Can you work these out from the model? Positions are in its coordinate system, mm. Face numbers are marked on the shaded views. Coordinates: 2 decimals unless noted, no trailing zeros. Order: outer loops, then holes, each group sorted by start corner. A loop starts at its lowest first (then second) coordinate and runs counter-clockwise, first axis right, second up. Notation, with made-up numbers: (-19, 47.5) -> (6, 47.5) arc R22 cw to (6, 64.5) -> close; hole circle Ø7 at (83.25, -12.5). An arc over 180 degrees is marked (long way). Return JSON: item names as keys, results as strings. Group by question number.
1) If we section it at C-C, the plane y = 7.25: Please give me the cut outline in (x, z) (3 decimals).
2) Thinking about a two-plate mould opening in Z: for the marked faces 1 and 2, which applies, +Z half, -Z half, draft (parallel to the pull), parting line (faces both ways), or undercut?
3) If I drill on probe 1 along Y at (x, z) = (-45.5, -2); probe 2 along Z at (x, y) = (-39, -1); probe 3 along Z at (x, y) = (-16, 0), over which ranges is the centre line in solid material (lowest first)? Write a range as from..to.
4) If we section it at B-B, the plane x = -43: Please give me the cut outline in (y, z), then the cut area to 3 significant figures.
5) For pin 1 (2 mm diameter, centred on y = -0.5, z = 1.5, fed in from +X); pin 2 (6 mm diameter, centred on x = -14, y = -0.5, fed in from -Z); pin 3 (1.5 mm diameter, centred on y = 2, z = -3, fed in from -X), each with a flat end and sliding along its axis, tell me the tip position at first contact or that it passes through.
from build123d import *

# Parameters (mm, degrees)
REVOLVE1_ANGLE                  = 67
BOSS_EXTRUDE1_REACH             = 76.037
BOSS_EXTRUDE1_END_RADIUS        = 72.791303716
BOSS_EXTRUDE1_DIRECTION_2_DEPTH = 4.5
BOSS_EXTRUDE2_DEPTH             = 4
BOSS_EXTRUDE3_DEPTH             = 1.35
CHAMFER1_SIZE                   = 0.5
SKETCH5_R                       = 1.475
BOSS_EXTRUDE4_DEPTH             = 7.1
SKETCH6_R                       = 3
BOSS_EXTRUDE5_DEPTH             = 3
BOSS_EXTRUDE5_TAPER             = 11
CHAMFER2_SIZE                   = 0.5
CHAMFER2_SIZE_2                 = 0.632256576


with BuildPart() as part:
    # Sketch1 → Revolve1 (revolve, symmetric)
    with BuildSketch(Plane.XY) as revolve1_sk:
        with BuildLine():
            Line((-60, 5), (-60.791303716, 5))
            Line((-60.791303716, 5), (-60.791303716, 6))
            Line((-60.791303716, 6), (-57.791303716, 6))
            Line((-57.791303716, 6), (-57.791303716, -6))
            Line((-57.791303716, -6), (-60.791303716, -6))
            Line((-60.791303716, -6), (-60.791303716, -5))
            Line((-60.791303716, -5), (-60, -5))
            ThreePointArc((-60, -5), (-59.791303716, 0), (-60, 5))
        make_face()
    revolve(axis=Axis((15, 24.442446043, 0), (0, -1, 0)), revolution_arc=REVOLVE1_ANGLE / 2)
    revolve(revolve1_sk.sketch, axis=Axis((15, 24.442446043, 0), (0, 1, 0)), revolution_arc=REVOLVE1_ANGLE / 2)

    # Boss-Extrude1: up to this cylinder (the profile starts inside it)
    boss_extrude1_end = Plane(origin=(15, 0, 0), z_dir=(0, 1, 0)) * Cylinder(BOSS_EXTRUDE1_END_RADIUS, 298.656607431, mode=Mode.PRIVATE)
    # Sketch2 → Boss-Extrude1 (add, up to the surface)
    with BuildSketch(Plane(origin=(0, 0, 0), x_dir=(0, 0, -1), z_dir=(1, 0, 0)), mode=Mode.PRIVATE) as boss_extrude1_sk1:
        with BuildLine():
            Line((2.75, 1.35), (-2.75, 1.35))
            ThreePointArc((-2.75, 1.35), (-2.926776695, 1.276776695), (-3, 1.1))
            Line((-3, 1.1), (-3, 1))
            ThreePointArc((-3, 1), (-2.926776695, 0.823223305), (-2.75, 0.75))
            Line((-2.75, 0.75), (-1.75, 0.75))
            ThreePointArc((-1.75, 0.75), (-1.573223305, 0.676776695), (-1.5, 0.5))
            Line((-1.5, 0.5), (-1.5, -0.5))
            ThreePointArc((-1.5, -0.5), (-1.573223305, -0.676776695), (-1.75, -0.75))
            Line((-1.75, -0.75), (-2.75, -0.75))
            ThreePointArc((-2.75, -0.75), (-2.926776695, -0.823223305), (-3, -1))
            Line((-3, -1), (-3, -1.1))
            ThreePointArc((-3, -1.1), (-2.926776695, -1.276776695), (-2.75, -1.35))
            Line((-2.75, -1.35), (2.75, -1.35))
            ThreePointArc((2.75, -1.35), (2.926776695, -1.276776695), (3, -1.1))
            Line((3, -1.1), (3, -1))
            ThreePointArc((3, -1), (2.926776695, -0.823223305), (2.75, -0.75))
            Line((2.75, -0.75), (1.75, -0.75))
            ThreePointArc((1.75, -0.75), (1.573223305, -0.676776695), (1.5, -0.5))
            Line((1.5, -0.5), (1.5, 0.5))
            ThreePointArc((1.5, 0.5), (1.573223305, 0.676776695), (1.75, 0.75))
            Line((1.75, 0.75), (2.75, 0.75))
            ThreePointArc((2.75, 0.75), (2.926776695, 0.823223305), (3, 1))
            Line((3, 1), (3, 1.1))
            ThreePointArc((3, 1.1), (2.926776695, 1.276776695), (2.75, 1.35))
        make_face()
    boss_extrude1_tool1 = extrude(boss_extrude1_sk1.sketch, amount=-BOSS_EXTRUDE1_REACH, mode=Mode.PRIVATE) & boss_extrude1_end
    add(boss_extrude1_tool1.solids().sort_by_distance((0, 0, 0))[0])

    # Sketch2 → Boss-Extrude1 direction 2 (add)
    with BuildSketch(Plane(origin=(0, 0, 0), x_dir=(0, 0, -1), z_dir=(1, 0, 0))):
        with BuildLine():
            Line((2.75, 1.35), (-2.75, 1.35))
            ThreePointArc((-2.75, 1.35), (-2.926776695, 1.276776695), (-3, 1.1))
            Line((-3, 1.1), (-3, 1))
            ThreePointArc((-3, 1), (-2.926776695, 0.823223305), (-2.75, 0.75))
            Line((-2.75, 0.75), (-1.75, 0.75))
            ThreePointArc((-1.75, 0.75), (-1.573223305, 0.676776695), (-1.5, 0.5))
            Line((-1.5, 0.5), (-1.5, -0.5))
            ThreePointArc((-1.5, -0.5), (-1.573223305, -0.676776695), (-1.75, -0.75))
            Line((-1.75, -0.75), (-2.75, -0.75))
            ThreePointArc((-2.75, -0.75), (-2.926776695, -0.823223305), (-3, -1))
            Line((-3, -1), (-3, -1.1))
            ThreePointArc((-3, -1.1), (-2.926776695, -1.276776695), (-2.75, -1.35))
            Line((-2.75, -1.35), (2.75, -1.35))
            ThreePointArc((2.75, -1.35), (2.926776695, -1.276776695), (3, -1.1))
            Line((3, -1.1), (3, -1))
            ThreePointArc((3, -1), (2.926776695, -0.823223305), (2.75, -0.75))
            Line((2.75, -0.75), (1.75, -0.75))
            ThreePointArc((1.75, -0.75), (1.573223305, -0.676776695), (1.5, -0.5))
            Line((1.5, -0.5), (1.5, 0.5))
            ThreePointArc((1.5, 0.5), (1.573223305, 0.676776695), (1.75, 0.75))
            Line((1.75, 0.75), (2.75, 0.75))
            ThreePointArc((2.75, 0.75), (2.926776695, 0.823223305), (3, 1))
            Line((3, 1), (3, 1.1))
            ThreePointArc((3, 1.1), (2.926776695, 1.276776695), (2.75, 1.35))
        make_face()
    extrude(amount=BOSS_EXTRUDE1_DIRECTION_2_DEPTH)

    # Sketch3 → Boss-Extrude2 (add, symmetric)
    with BuildSketch(Plane(origin=(0, 0, 0), x_dir=(1, 0, 0), z_dir=(0, 1, 0))):
        with BuildLine():
            Line((-55.656379023, 17.5), (-55.656379023, -17.5))
            ThreePointArc((-55.656379023, -17.5), (-57.791303716, 0), (-55.656379023, 17.5))
        make_face()
    extrude(amount=BOSS_EXTRUDE2_DEPTH, both=True)

    # Sketch4 → Boss-Extrude3 (add, symmetric)
    with BuildSketch(Plane(origin=(0, 0, 0), x_dir=(1, 0, 0), z_dir=(0, 1, 0))):
        Polygon((-55.656379023, -12.5), (-55.656379023, 12.5), (-48.656379023, 0), align=None)
    extrude(amount=BOSS_EXTRUDE3_DEPTH, both=True)

    # Chamfer1
    chamfer1_edges = [part.edges().sort_by_distance(p)[0] for p in [
        (-55.656379023, -4, 0),
        (-55.656379023, 4, 0),
    ]]
    chamfer(chamfer1_edges, length=CHAMFER1_SIZE)

    # Sketch5 → Boss-Extrude4 (add)
    with BuildSketch(Plane(origin=(0, 1.35, 0), x_dir=(1, 0, 0), z_dir=(0, 1, 0))):
        with Locations(Location((1.8, 0, 0), (0, 0, 90))):
            Circle(SKETCH5_R)
    extrude(amount=BOSS_EXTRUDE4_DEPTH)

    # Sketch6 → Boss-Extrude5 (add)
    with BuildSketch(Plane(origin=(0, 8.45, 0), x_dir=(1, 0, 0), z_dir=(0, 1, 0))):
        with Locations((1.8, 0)):
            Circle(SKETCH6_R)
    extrude(amount=BOSS_EXTRUDE5_DEPTH, taper=BOSS_EXTRUDE5_TAPER)

    # Chamfer2
    # the kernel refuses this chamfer: 0.632256576, 0.5 mm, written as the material it takes off along each edge
    with BuildSketch(Plane(origin=(1.8, 11.45, 0), x_dir=(1, 0, 0), z_dir=(0, 0, -1))) as chamfer2_piece_1:
        Polygon((2.416859073 + CHAMFER2_SIZE * 0.190808995377, CHAMFER2_SIZE * 0.981627183448), (2.416859073 - CHAMFER2_SIZE_2, 0), (2.416859073, 0), align=None)
    revolve(axis=Axis((1.8, 11.45, 0), (0, -1, 0)), mode=Mode.SUBTRACT)


solid = part.part
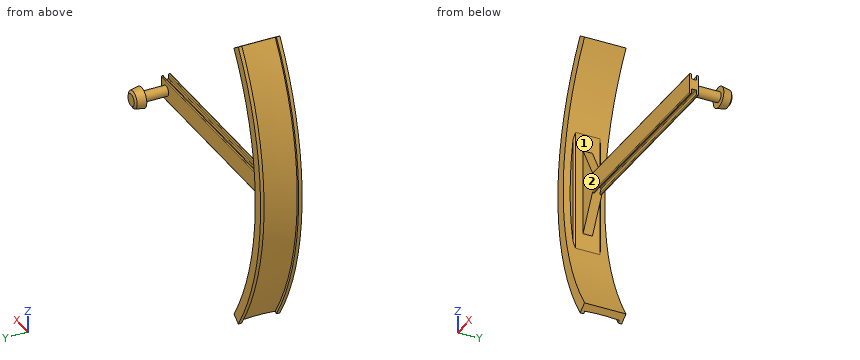
Result sheet:
{
 "1": {"outline": "circle Ø2.95 at (1.8, 0)"},
 "2": {"face 1": "undercut", "face 2": "undercut"},
 "3": {"probe 1": "y = -1.35..-0.75, 0.75..1.35", "probe 2": "z = -3..3", "probe 3": "z = -1.5..1.5"},
 "4": {"outline": "(-1.35, -2.75) arc R0.25 ccw to (-1.1, -3) -> (-1, -3) arc R0.25 ccw to (-0.75, -2.75) -> (-0.75, -1.75) arc R0.25 cw to (-0.5, -1.5) -> (0.5, -1.5) arc R0.25 cw to (0.75, -1.75) -> (0.75, -2.75) arc R0.25 ccw to (1, -3) -> (1.1, -3) arc R0.25 ccw to (1.35, -2.75) -> (1.35, 2.75) arc R0.25 ccw to (1.1, 3) -> (1, 3) arc R0.25 ccw to (0.75, 2.75) -> (0.75, 1.75) arc R0.25 cw to (0.5, 1.5) -> (-0.5, 1.5) arc R0.25 cw to (-0.75, 1.75) -> (-0.75, 2.75) arc R0.25 ccw to (-1, 3) -> (-1.1, 3) arc R0.25 ccw to (-1.35, 2.75) -> close", "area": "11.6 mm2"},
 "5": {"pin 1": "stops at x = 4.5", "pin 2": "stops at z = -3", "pin 3": "stops at x = -59.8"}
}
